Autodesk Inventor part; units mm, degrees
ref_plane "YZ Plane" through (0, 0, 0) normal (1, 0, 0) x (0, 1, 0)
ref_plane "XZ Plane" through (0, 0, 0) normal (0, 1, 0) x (-1, 0, 0)
ref_plane "XY Plane" through (0, 0, 0) normal (0, 0, 1) x (1, 0, 0)
sketch "Skizze1" plane through (0, 0, 0) normal (0, 1, 0) x (-1, 0, 0)
  line L0 (7.5, 16.5) -> (0, 16.5)
  line L1 (0, 16.5) -> (0, -16.5)
  line L2 (0, -16.5) -> (7.5, -16.5)
  line L3 (10.5, -13.5) -> (10.5, 13.5)
  circle A0 centre (5.25, 8.25) radius 3.25
  line L4 (10.5, 0) -> (0, 0) construction
  circle A1 centre (5.25, -8.25) radius 3.25
  arc A2 (10.5, 13.5) -> (7.5, 16.5) centre (7.5, 13.5) ccw
  arc A3 (7.5, -16.5) -> (10.5, -13.5) centre (7.5, -13.5) ccw
  point P0 (5.25, 0)
  dimension "d0" = 2
  dimension "d1" = 6.5
  dimension "d2" = 5
  dimension "d3" = 10
  dimension "d4" = 3
extrude "Extrusion1" add sketch "Skizze1" along normal blind 4
sketch "Skizze3" plane through (0, 0, 16.5) normal (1, 0, 0) x (0, 0, -1)
  line L0 (0, 0) -> (33, 0)
  line L1 (33, 0) -> (0, 0)
  line L2 (0, 0) -> (0, 16)
  line L3 (0, 16) -> (33, 16)
  line L4 (33, 16) -> (33, 0)
  point P0 (16.5, 0)
  point P1 (33, 4)
  dimension "d21" = 12
extrude "Extrusion2" add sketch "Skizze3" along normal blind 6
sketch "Skizze4" plane through (0, 0, 16.5) normal (-1, 0, 0) x (0, 0, 1)
  point P0 (-16.5, 0)
sketch "Skizze5" plane through (0, 0, 16.5) normal (-1, 0, 0) x (0, 0, 1)
  line L0 (0, 4) -> (-33, 4)
  line L1 (0, 16) -> (0, 4)
  line L2 (-33, 16) -> (0, 16)
  line L3 (-33, 4) -> (-33, 16)
  line L4 (-33, 16) -> (0, 16) construction
  line L5 (-16.5, 16) -> (-16.5, 4) construction
  line L6 (-30, 4) -> (-3, 4) construction
  line L7 (-16.5, 10) -> (-33, 10) construction
  line L8 (-33, 0) -> (-33, 16) construction
  point P0 (-16.5, 0)
  point P1 (-24.75, 10)
  point P2 (-8.25, 10)
  point P3 (-24.75, 10)
hole "Bohrung1" at (0, 10, 8.25) at (0, 10, -8.25) direction (1, 0, 0) diameter 5 end through all countersink diameter 8.6 countersink angle 90
fillet "Rundung1" radius 2 1 edges at (0, 4, 0)
fillet "Rundung2" radius 4 2 edges at (3, 16, 16.5) (3, 16, -16.5)
fillet "Rundung3" radius 0.5 22 edges at (6, 14.8284, 15.3284) (6, 16, 0) (6, 14.8284, -15.3284) (6, 6, -16.5) (6, 6, 16.5) (-9.6213, 0, 15.6213) (-10.5, 0, 0) (-9.6213, 0, -15.6213) (-0.75, 0, -16.5) (-0.75, 0, 16.5) (0, 9, 16.5) (-0.5858, 4.5858, 16.5) (-4.75, 4, 16.5) (-9.6213, 4, 15.6213) (-10.5, 4, 0) (-9.6213, 4, -15.6213) (-4.75, 4, -16.5) (-0.5858, 4.5858, -16.5) (0, 9, -16.5) (0, 14.8284, -15.3284) (0, 16, 0) (0, 14.8284, 15.3284)
sketch "Skizze7" plane through (0, 4, 0) normal (0, 1, 0) x (1, 0, 0)
  circle A0 centre (-5.25, -8.25) radius 3.25
  circle A1 centre (-5.25, 8.25) radius 3.25
  circle A2 centre (-5.25, -8.25) radius 5.25
  circle A3 centre (-5.25, 8.25) radius 5.25
  point P0 (0, 0)
  point P1 (-2, -8.25)
  point P2 (-2, 8.25)
  dimension "d32" = 2
extrude "Extrusion3" cut sketch "Skizze7" along normal up to surface (12 mm away)
properties part number "Wlan-antennen-halter"
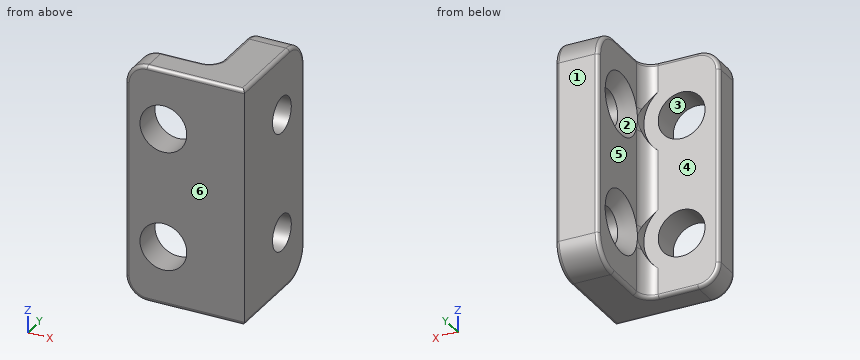
Verification items for the finished model (mm, model axes). Face numbers are marked on the shaded views. A direction names the side the tool comes from. Coordinates: 2 decimals unless noted, no trailing zeros. Order: outer loops, then holes, each group sorted by start corner. A loop starts at its lowest first (then second) coordinate and runs counter-clockwise, first axis right, second up. Notation, with made-up numbers: M -27,-8.75 L 8,-8.75 A20 cw 8,3.25 Z; hole C 45.5,81.5 d9. An arc over 180 degrees is marked long. One line per item, written item: value. Start each with the question number.
Item 1: Sectioned sample at A-A (y = 10). Enter the section's corners in (x, z), then the cut area to 3 significant figures.
Item 2: Sectioned sample at C-C (z = 1). Enter the section's corners in (x, y).
Item 3: Sectioned sample at B-B (x = -5.25). Enter the section's corners in (y, z).
Item 4: Sectioned sample at D-D (y = 2). Enter the section's corners in (x, z), then the cut area to 3 significant figures.
Item 5: Access from +Z, -Z, +X, -X, +Y, -Y to the whole of each face (thin tool, end or side, straight path). Record for the marked faces 4, 5 and 6.
Item 6: Scan lines: probe 1 along Z at (x, y) = (-5.25, 1.65); probe 2 along Z at (x, y) = (3.5, 10); probe 3 along Y at (x, z) = (3.9, -8.25). Record each from-to range of solid material in increasing order.
Item 7: Mould release check, pull along Y, two halves, no side actions. Record for the marked faces 1, 2 and 3: released by +Y, released by -Y, zero draft, split by the parting line, or undercut.
Item 8: Gauge pin test, flat ends, axial feed: pin 1 (6 mm diameter, centred on y = 12, z = 12, fed in from -X); pin 2 (5 mm diameter, centred on x = -3.5, z = 6.5, fed in from +Y). Record the tip position at first contact, or that the pin passes through.
Conclusion:
1. outline: M 0,-16 A0.5 ccw 0.5,-16.5 L 5.5,-16.5 A0.5 ccw 6,-16 L 6,-10.75 L 1.8,-10.75 L 0,-12.55 Z; M 0,-3.95 L 1.8,-5.75 L 6,-5.75 L 6,5.75 L 1.8,5.75 L 0,3.95 Z; M 0,12.55 L 1.8,10.75 L 6,10.75 L 6,16 A0.5 ccw 5.5,16.5 L 0.5,16.5 A0.5 ccw 0,16 Z
1. area: 131 mm^2
2. outline: M -10.5,0.5 A0.5 ccw -10,0 L 6,0 L 6,15.5 A0.5 ccw 5.5,16 L 0.5,16 A0.5 ccw 0,15.5 L 0,6 A2 cw -2,4 L -10,4 A0.5 ccw -10.5,3.5 Z
3. outline: M 0,-16 A0.5 ccw 0.5,-16.5 L 3.5,-16.5 A0.5 ccw 4,-16 L 4,-11.5 L 0,-11.5 Z; M 0,-5 L 4,-5 L 4,5 L 0,5 Z; M 0,11.5 L 4,11.5 L 4,16 A0.5 ccw 3.5,16.5 L 0.5,16.5 A0.5 ccw 0,16 Z
4. outline: M -10.5,-13.5 A3 ccw -7.5,-16.5 L 5.5,-16.5 A0.5 ccw 6,-16 L 6,16 A0.5 ccw 5.5,16.5 L -7.5,16.5 A3 ccw -10.5,13.5 Z; hole C -5.25,-8.25 d6.5; hole C -5.25,8.25 d6.5
4. area: 474 mm^2
5. face 4: -X, +Y
5. face 5: +Z, -Z, -X, +Y
5. face 6: +Z, -Z, +X, -X, -Y
6. probe 1: z = -16.5 to -11.5, -5 to 5, 11.5 to 16.5
6. probe 2: z = -16.5 to -10.75, -5.75 to 5.75, 10.75 to 16.5
6. probe 3: y = 0 to 7.5, 12.5 to 16
7. face 1: released by +Y
7. face 2: undercut
7. face 3: zero draft
8. pin 1: stops at x = 0
8. pin 2: stops at y = 4
